from build123d import *

# Parameters (mm, degrees)
SKETCH1_W             = 25
SKETCH1_H             = 25
BASE_PLATE_DEPTH      = 3
M2X0_4_TAPPED_HOLE1_D = 1.6
SKETCH6_W             = 12
SKETCH6_H             = 12
LENSE_BASE_DEPTH      = 10


# Read off the part's stored shape, not the designer's step: lense
with BuildPart() as part:
    # Sketch1 → base_plate (new body)
    with BuildSketch(Plane(origin=(0, 0, 0), x_dir=(1, 0, 0), z_dir=(0, 1, 0))):
        Rectangle(SKETCH1_W, SKETCH1_H)
    extrude(amount=BASE_PLATE_DEPTH)

    # M2x0.4 Tapped Hole1 (through all)
    with Locations(Plane(origin=(-11, 3, -3), x_dir=(0, 0, 1), z_dir=(0, 1, 0))):
        with Locations((0, 0), (14, 0), (14, 22), (0, 22)):
            Hole(M2X0_4_TAPPED_HOLE1_D / 2)

    # Sketch6 → lense_base (add)
    with BuildSketch(Plane(origin=(0, 3, 0), x_dir=(1, 0, 0), z_dir=(0, 1, 0))):
        with Locations((0, 3)):
            Rectangle(SKETCH6_W, SKETCH6_H)
    extrude(amount=LENSE_BASE_DEPTH)

    # lense outline → lense (revolve)
    with BuildSketch(Plane.XY.offset(-3)):
        with BuildLine():
            Line((0, 12.999999997), (3.500000006, 12.999999997))
            ThreePointArc((3.500000006, 12.999999997), (1.820027476, 13.745096152), (0, 14))
            Line((0, 14), (0, 12.999999997))
        make_face()
    revolve(axis=Axis((0, 0, -3), (0, 1, 0)))


solid = part.part
CAD build for the part. Positions are in the model's coordinates, mm. A direction names the side the tool comes from. Coordinates: 2 decimals unless noted, no trailing zeros. Write each loop counter-clockwise with the first axis right and the second up, starting at its lowest first coordinate (ties: lowest second). Pieces come first, ordered by that corner, then holes. Notation, with made-up numbers: (46.25, 2.25) - (65.25, 2.25) arc R19 cw to (65.25, 25.25) - close; hole circle Ø3 at (0, 26.25). An arc over 180 degrees is marked (long way). Use a Markdown table: item, result. Add a question column.
Item 1: Band-saw the part on C-C, the plane z = 2.5. Give the cut face in (x, y), and give its area (3 significant figures).
Item 2: Band-saw the part on D-D, the plane z = -3. Give the cut face in (x, y) (3 decimals).
Item 3: Band-saw the part on B-B, the plane z = 11. Give the cut face in (x, y).
Item 4: 3-axis set-ups, long thin cutter, end or side, ignore diameter. For faces 1 (the face through (-6, 8, -3)), 2 (the face through (6, 8, -3)), 3 (the face through (0, 8, 3)): which of +Z, -Z, +X, -X, +Y, -Y reach the whole face in a straight line?
Item 5: Mould opens along X. For faces 4 (the face through (-10.207, 1.479, 11.104)), 5 (the face through (12.5, 1, 0)), 6 (the face through (0, 8, -9)), 7 (the face through (-12.5, 1, 0)) say: pulls with the +X half, pulls with the -X half, needs draft (parallel to the pull), parting line crosses it, or undercut.
Item 6: Band-saw the part on A-A, the plane x = 11. Give the cut face in (y, z), and give its area (3 significant figures).
Item 7: Flat gauge pins, fed straight in: pin 1 (5 mm diameter, centred on y = 11.5, z = -2.5, fed in from -X); pin 2 (8 mm diameter, centred on y = 8, z = -6.5, fed in from +X); pin 3 (3 mm diameter, centred on x = -6, y = 11, fed in from +Z). Where does each tip first touch, or does it go through?
Item 8: Drill centre lines: L1, parallel to X at y = 1.3, z = -3; L2, parallel to X at y = 10.25, z = -6.5; L3, parallel to Y at x = 10.25, z = 10. Where is each one in solid material? Low to high. Write a range as from..to.
Numbers:
| question | item | result |
|---|---|---|
| 1 | outline | (-12.5, 0) - (12.5, 0) - (12.5, 3) - (6, 3) - (6, 13) - (-6, 13) - (-6, 3) - (-12.5, 3) - close |
| 1 | area | 195 mm2 |
| 2 | outline | (-12.5, 0) - (-11.8, 0) - (-11.8, 3) - (-12.5, 3) - close; (-10.2, 0) - (10.2, 0) - (10.2, 3) - (6, 3) - (6, 13) - (3.5, 13) arc R6.625 ccw to (-3.5, 13) - (-6, 13) - (-6, 3) - (-10.2, 3) - close; (11.8, 0) - (12.5, 0) - (12.5, 3) - (11.8, 3) - close |
| 3 | outline | (-12.5, 0) - (-11.8, 0) - (-11.8, 3) - (-12.5, 3) - close; (-10.2, 0) - (10.2, 0) - (10.2, 3) - (-10.2, 3) - close; (11.8, 0) - (12.5, 0) - (12.5, 3) - (11.8, 3) - close |
| 4 | face 1 | +Z, -Z, -X, +Y |
| 4 | face 2 | +Z, -Z, +X, +Y |
| 4 | face 3 | +Z, +X, -X, +Y |
| 5 | face 4 | undercut |
| 5 | face 5 | pulls with the +X half |
| 5 | face 6 | needs draft |
| 5 | face 7 | pulls with the -X half |
| 6 | outline | (0, -12.5) - (3, -12.5) - (3, -3.8) - (0, -3.8) - close; (0, -2.2) - (3, -2.2) - (3, 10.2) - (0, 10.2) - close; (0, 11.8) - (3, 11.8) - (3, 12.5) - (0, 12.5) - close |
| 6 | area | 65.4 mm2 |
| 7 | pin 1 | x = -6 |
| 7 | pin 2 | x = 6 |
| 7 | pin 3 | z = 3 |
| 8 | L1 | -12.5..-11.8, -10.2..10.2, 11.8..12.5 |
| 8 | L2 | -6..6 |
| 8 | L3 | 0..3 |
